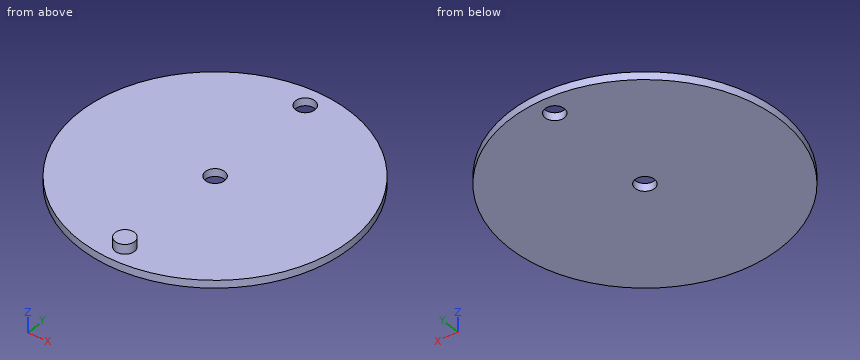
```python
from build123d import *

# Parameters (mm, degrees)
SKETCH1_R           = 88.9
SKETCH1_R_2         = 6.35
BOSS_EXTRUDE1_DEPTH = 5.08
SKETCH2_R           = 6.35
BOSS_EXTRUDE2_DEPTH = 11.43


with BuildPart() as part:
    # Sketch1 → Boss-Extrude1 (new body)
    with BuildSketch(Plane.XY):
        Circle(SKETCH1_R)
        Circle(SKETCH1_R_2, mode=Mode.SUBTRACT)
        with Locations((0, -76.2)):
            Circle(SKETCH1_R_2, mode=Mode.SUBTRACT)
        with Locations((0, 76.2)):
            Circle(SKETCH1_R_2, mode=Mode.SUBTRACT)
    extrude(amount=BOSS_EXTRUDE1_DEPTH)

    # Sketch2 → Boss-Extrude2 (add)
    with BuildSketch(Plane.XY):
        with Locations((0, -76.2)):
            Circle(SKETCH2_R)
    extrude(amount=BOSS_EXTRUDE2_DEPTH)


solid = part.part
```
The listing builds one solid part. Answer for the finished solid, in the listing's coordinates (mm). Give positions to 0.01 mm unless a question says otherwise; leave off trailing zeros. Loops run counter-clockwise (first coordinate to the right, second up) from the corner with the lowest first, then second, coordinate; pieces in that order, holes last. Notation, with made-up numbers: M 66,16.5 L 93,16.5 A20 cw 93,25.5 Z; hole C -9.75,47.25 d8. An arc over 180 degrees is marked long. One line per item, written item: value.
Q1. A cutting plane is placed at C-C on y = -76.2. Determine the outline of the cut face in (x, z), then the cut area to 3 significant figures.
Working result:
outline: M -45.79,0 L 45.79,0 L 45.79,5.08 L 6.35,5.08 L 6.35,11.43 L -6.35,11.43 L -6.35,5.08 L -45.79,5.08 Z
area: 546 mm^2
Q2. A cutting plane is placed at D-D on x = 70. Determine the outline of the cut face in (y, z).
Working result:
outline: M -54.8,0 L 54.8,0 L 54.8,5.08 L -54.8,5.08 Z
Q3. Flat-ended cylindrical pins translate along their axes: P1, Ø1.5, axis at x = 19.5, z = 5.5, coming from the -Y side; P2, Ø5, axis at y = -53, z = 1.5, coming from the +X side; P3, Ø16.5, axis at x = 0, y = 0, coming from the +Z side. Find the tip coordinate at first contact, or state that the pin passes through.
Working result:
P1: stops at y = -86.87
P2: stops at x = 73.16
P3: stops at z = 5.08
Q4. A cutting plane is placed at A-A on x = 0. Determine the outline of the cut face in (y, z).
Working result:
outline: M -88.9,0 L -6.35,0 L -6.35,5.08 L -69.85,5.08 L -69.85,11.43 L -82.55,11.43 L -82.55,5.08 L -88.9,5.08 Z; M 6.35,0 L 69.85,0 L 69.85,5.08 L 6.35,5.08 Z; M 82.55,0 L 88.9,0 L 88.9,5.08 L 82.55,5.08 Z
Q5. Find the intervals of material crossed by line 1 (Y direction, x = 0, z = 1.7); line 2 (Z direction, x = 34.5, y = 35.5); line 3 (X direction, y = 2, z = 2.5), in increasing order. Write a range as from..to.
Working result:
line 1: y = -88.9..-6.35, 6.35..69.85, 82.55..88.9
line 2: z = 0..5.08
line 3: x = -88.88..-6.03, 6.03..88.88
Q6. A cutting plane is placed at B-B on y = 0. Determine the outline of the cut face in (x, z).
Working result:
outline: M -88.9,0 L -6.35,0 L -6.35,5.08 L -88.9,5.08 Z; M 6.35,0 L 88.9,0 L 88.9,5.08 L 6.35,5.08 Z
